Source: three-view drawing plus pictorial views. Frame: mm from the lowest corner of the part. A direction names the side the tool comes from. Give positions to 0.01 mm unless a question says otherwise; leave off trailing zeros. Loops run counter-clockwise (first coordinate to the right, second up) from the corner with the lowest first, then second, coordinate; pieces in that order, holes last. Notation, with made-up numbers: (80.5, -25) -> (126.5, -25) arc R19 cw to (126.5, -6) -> close; hole circle Ø8 at (3, -8). An arc over 180 degrees is marked (long way). Answer in a Markdown table with one row per item. Add a question column.
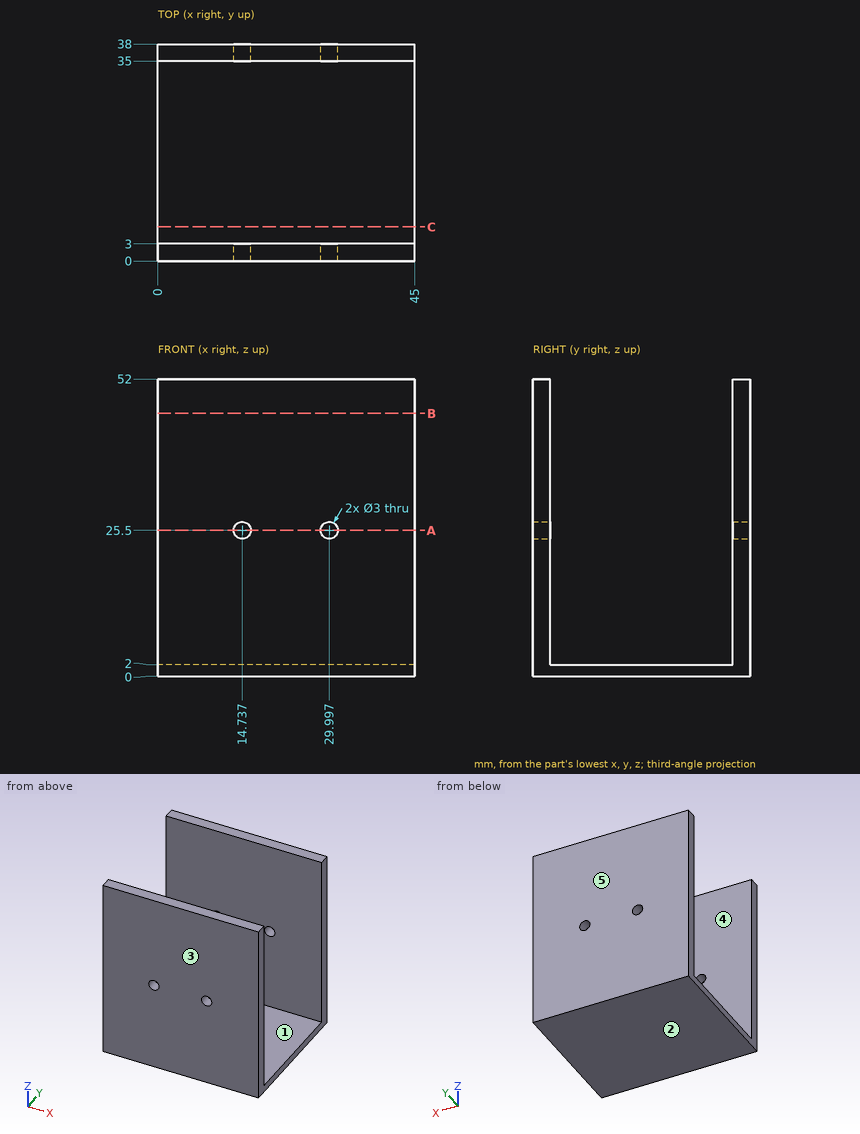
(1) Material intervals for line 1 along X through (y, z) = (36.55, 25.5); line 2 along Y through (x, z) = (38.5, 13.5); line 3 along X through (y, z) = (37, 25), sorted ascending. Write a range as from..to.
(2) Cut plane C-C on y = 6. Return the cut outline in (x, z), then the cut area to 3 significant figures.
(3) Pin query (flat end, axial travel): pin 1 Ø2.5 at (x, z) = (14.737, 25.5) entering from +Y. Return the tip coordinate at first contact, or that it passes through.
(4) Cut plane A-A on z = 25.5. Return the cut outline in (x, y).
(5) Draft query along Y for the marked faces 1, 2 and 3. Return one class per face: +Y half, -Y half, draft (parallel to the pull), parting line (faces both ways), or undercut.
(6) Cut plane B-B on z = 46. Return the cut outline in (x, y).
(7) Reachability of the marked faces 4 and 5 from +Z, -Z, +X, -X, +Y, -Y: full face, straight path, thin tool, end or side. Return the list, or none.
Answer list:
| question | item | result |
|---|---|---|
| 1 | line 1 | x = 0..13.24, 16.24..28.5, 31.5..45 |
| 1 | line 2 | y = 0..3, 35..38 |
| 1 | line 3 | x = 0..13.32, 16.15..28.58, 31.41..45 |
| 2 | outline | (0, 0) -> (45, 0) -> (45, 2) -> (0, 2) -> close |
| 2 | area | 90.0 mm² |
| 3 | pin 1 | passes through |
| 4 | outline | (0, 0) -> (13.24, 0) -> (13.24, 3) -> (0, 3) -> close; (0, 35) -> (13.24, 35) -> (13.24, 38) -> (0, 38) -> close; (16.24, 0) -> (28.5, 0) -> (28.5, 3) -> (16.24, 3) -> close; (16.24, 35) -> (28.5, 35) -> (28.5, 38) -> (16.24, 38) -> close; (31.5, 0) -> (45, 0) -> (45, 3) -> (31.5, 3) -> close; (31.5, 35) -> (45, 35) -> (45, 38) -> (31.5, 38) -> close |
| 5 | face 1 | undercut |
| 5 | face 2 | draft |
| 5 | face 3 | -Y half |
| 6 | outline | (0, 0) -> (45, 0) -> (45, 3) -> (0, 3) -> close; (0, 35) -> (45, 35) -> (45, 38) -> (0, 38) -> close |
| 7 | face 4 | +Z, +X, -X |
| 7 | face 5 | +Z, -Z, +X, -X, +Y |
